from build123d import *

# Parameters (mm, degrees)
BOSS_EXTRUDE1_DEPTH = 3
SKETCH2_R           = 16
BOSS_EXTRUDE2_DEPTH = 32
SKETCH3_R           = 13.8
BOSS_EXTRUDE3_DEPTH = 38
SKETCH4_R           = 18
SKETCH4_R_2         = 13.8
BOSS_EXTRUDE4_DEPTH = 17
SKETCH6_R           = 1.5
CUT_EXTRUDE1_DEPTH  = 10


with BuildPart() as part:
    # Sketch1 → Boss-Extrude1 (new body)
    with BuildSketch(Plane.XY):
        with BuildLine():
            Line((-4.002811512, 9), (4.002811512, 9))
            ThreePointArc((4.002811512, 9), (9.85, 0), (4.002811512, -9))
            Line((4.002811512, -9), (-4.002811512, -9))
            ThreePointArc((-4.002811512, -9), (-9.85, 0), (-4.002811512, 9))
        make_face()
    extrude(amount=BOSS_EXTRUDE1_DEPTH)

    # Sketch2 → Boss-Extrude2 (add)
    with BuildSketch(Plane(origin=(0, 0, 0), x_dir=(-1, 0, 0), z_dir=(0, 0, -1))):
        Circle(SKETCH2_R)
    extrude(amount=BOSS_EXTRUDE2_DEPTH)

    # Sketch3 → Boss-Extrude3 (add)
    with BuildSketch(Plane(origin=(0, 0, -32), x_dir=(-1, 0, 0), z_dir=(0, 0, -1))):
        Circle(SKETCH3_R)
    extrude(amount=BOSS_EXTRUDE3_DEPTH)

    # Sketch4 → Boss-Extrude4 (add)
    with BuildSketch(Plane(origin=(0, 0, -70), x_dir=(-1, 0, 0), z_dir=(0, 0, -1))):
        Circle(SKETCH4_R)
        Circle(SKETCH4_R_2, mode=Mode.SUBTRACT)
        Circle(SKETCH4_R_2)
        with BuildLine():
            Line((-17.654073056, -3.511937432), (-30.0520382, -15.909902577))
            Line((-30.0520382, -15.909902577), (-15.909902577, -30.0520382))
            Line((-15.909902577, -30.0520382), (-3.511937432, -17.654073056))
            ThreePointArc((-3.511937432, -17.654073056), (-12.727922061, -12.727922061), (-17.654073056, -3.511937432))
        make_face()
    extrude(amount=BOSS_EXTRUDE4_DEPTH)

    # Sketch6 → Cut-Extrude1 (cut)
    with BuildSketch(Plane.XY):
        with Locations((-9.192388155, 9.192388155)):
            Circle(SKETCH6_R)
        with Locations((9.192388155, 9.192388155)):
            Circle(SKETCH6_R)
        with Locations((9.192388155, -9.192388155)):
            Circle(SKETCH6_R)
        with Locations((-9.192388155, -9.192388155)):
            Circle(SKETCH6_R)
    extrude(amount=-CUT_EXTRUDE1_DEPTH, mode=Mode.SUBTRACT)


solid = part.part
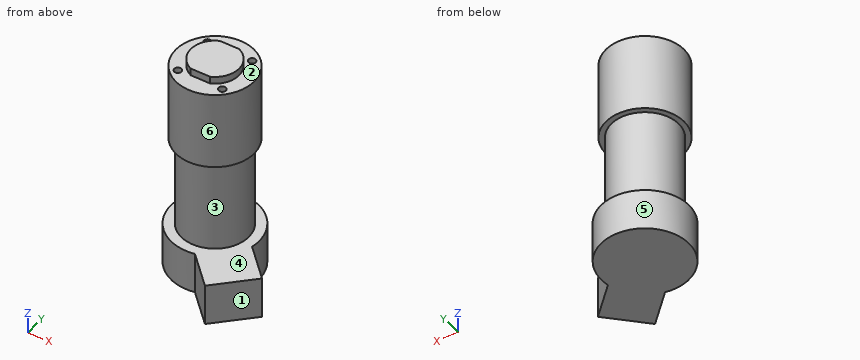
Read the model definition and answer for the solid it produces. Units are mm, in the model's axes. Face numbers are marked on the shaded views. A direction names the side the tool comes from. Coordinates: 2 decimals unless noted, no trailing zeros. Write each loop counter-clockwise with the first axis right and the second up, starting at its lowest first coordinate (ties: lowest second). Pieces come first, ordered by that corner, then holes. Notation, with made-up numbers: (-34.75, -8.5) -> (7.25, -8.5) arc R34 ccw to (7.25, 21.5) -> close; hole circle Ø6 at (7, 80.5). An arc over 180 degrees is marked (long way). Return JSON: item names as keys, results as strings.
(1) Each of these flat-tipped pins is pushed along its axis until it touches: P1, Ø3, axis at x = 8.5, z = -77.5, coming from the -Y side; P2, Ø4, axis at x = -9.19, y = -9.19, coming from the +Z side; P3, Ø0.9, axis at x = 8.5, y = 9, coming from the +Z side. Where does it stop, or does it pass through?
Answers below:
{"P1": "y = -24.14", "P2": "z = 0", "P3": "z = -10"}
(2) The part is cut by section C-C on z = -21. Give the vertices of the cut face in (x, y), then the cut area to 3 significant figures.
Answers below:
{"outline": "circle Ø32 at (0, 0)", "area": "804 mm^2"}
(3) For a pull along Z with two mould halves and no side action, classify the marked faces 1, 2, 3 and 4 as pulls with the +Z half, pulls with the -Z half, needs draft (parallel to the pull), parting line crosses it, or undercut.
Answers below:
{"face 1": "needs draft", "face 2": "pulls with the +Z half", "face 3": "undercut", "face 4": "undercut"}
(4) Which of the six approach directions +Z, -Z, +X, -X, +Y, -Y give full straight-line access (tool end or side, diameter ignored) to the marked faces 5 and 6?
Answers below:
{"face 5": "+Z, -Z", "face 6": "+Z"}
(5) The part is cut by section D-D on x = -12. Give the vertices of the cut face in (y, z), then the cut area to 3 significant figures.
Answers below:
{"outline": "(-13.42, -87) -> (13.42, -87) -> (13.42, -70) -> (6.81, -70) -> (6.81, -32) -> (10.58, -32) -> (10.58, 0) -> (-10.58, 0) -> (-10.58, -32) -> (-6.81, -32) -> (-6.81, -70) -> (-13.42, -70) -> close", "area": "1,650 mm^2"}
(6) The part is cut by section B-B on x = 0. Give the vertices of the cut face in (y, z), then the cut area to 3 significant figures.
Answers below:
{"outline": "(-18, -87) -> (18, -87) -> (18, -70) -> (13.8, -70) -> (13.8, -32) -> (16, -32) -> (16, 0) -> (9, 0) -> (9, 3) -> (-9, 3) -> (-9, 0) -> (-16, 0) -> (-16, -32) -> (-13.8, -32) -> (-13.8, -70) -> (-18, -70) -> close", "area": "2,740 mm^2"}
(7) The part is cut by section A-A on y = 0. Give the vertices of the cut face in (x, z), then the cut area to 3 significant figures.
Answers below:
{"outline": "(-18, -87) -> (18, -87) -> (18, -70) -> (13.8, -70) -> (13.8, -32) -> (16, -32) -> (16, 0) -> (9.85, 0) -> (9.85, 3) -> (-9.85, 3) -> (-9.85, 0) -> (-16, 0) -> (-16, -32) -> (-13.8, -32) -> (-13.8, -70) -> (-18, -70) -> close", "area": "2,740 mm^2"}
(8) Consider line 1 along Z through (x, y) = (-10, 2); line 2 along Z through (x, y) = (28, -14.5); line 3 along X through (y, z) = (-9, -4). Determine where each line is inside the solid, lowest interval first. Write a range as from..to.
Answers below:
{"line 1": "-87..0", "line 2": "-87..-70", "line 3": "-13.23..-10.68, -7.7..7.7, 10.68..13.23"}
